Design review of the part shown in the three views and the two pictorial views. Dimensions are in mm from the part's minimum x, y and z. Coordinates: 2 decimals unless noted, no trailing zeros. Loops run counter-clockwise (first coordinate to the right, second up) from the corner with the lowest first, then second, coordinate; pieces in that order, holes last. Notation, with made-up numbers: (86.25, 74.25) -> (143.25, 74.25) arc R13 ccw to (143.25, 99.25) -> close; hole circle Ø4 at (78.5, 32). An arc over 180 degrees is marked (long way). One line per item, written item: value. Start each with the question number.
1. Draft analysis for pull direction Z (two halves, no side actions). For the marked faces 1, 2 and 3, state which applies: pulls with the +Z half, pulls with the -Z half, needs draft (parallel to the pull), parting line crosses it, or undercut.
2. Add section D-D on z = 48.5. Write out the cut boundary in (x, y).
3. Add section A-A on x = 14. Write out the cut boundary in (y, z).
4. For probe 1 along X at (y, z) = (2.5, 47.75); probe 2 along Z at (x, y) = (14, 3.15); probe 3 along X at (y, z) = (4.05, 3.5), list the stretches that pass through material, from the lowest coordinate up.
5. Insertion check: pin 1 (3 mm diameter, centred on x = 24, y = 2.5, fed in from -Z); pin 2 (3 mm diameter, centred on x = 4, y = 2.5, fed in from +Z). Each pin has a flat end and moves straight along its axis. Give the tip position at first contact, or say it passes through.
6. Add section B-B on z = 24. Write out the cut boundary in (x, y).
7. Add section C-C on y = 2.5. Write out the cut boundary in (x, z).
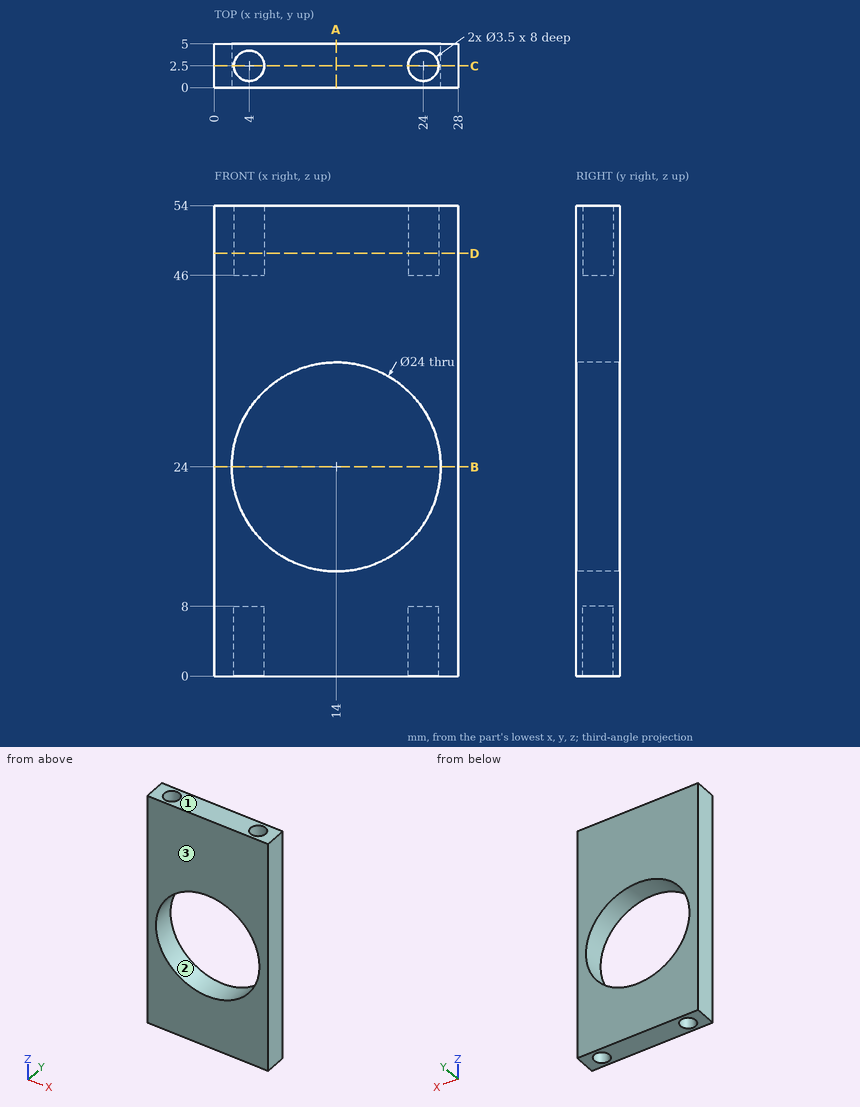
Worked answers:
1. face 1: pulls with the +Z half
1. face 2: undercut
1. face 3: needs draft
2. outline: (0, 0) -> (28, 0) -> (28, 5) -> (0, 5) -> close; hole circle Ø3.5 at (4, 2.5); hole circle Ø3.5 at (24, 2.5)
3. outline: (0, 0) -> (5, 0) -> (5, 12) -> (0, 12) -> close; (0, 36) -> (5, 36) -> (5, 54) -> (0, 54) -> close
4. probe 1: x = 0 to 2.25, 5.75 to 22.25, 25.75 to 28
4. probe 2: z = 0 to 12, 36 to 54
4. probe 3: x = 0 to 3.19, 4.81 to 23.19, 24.81 to 28
5. pin 1: stops at z = 8
5. pin 2: stops at z = 46
6. outline: (0, 0) -> (2, 0) -> (2, 5) -> (0, 5) -> close; (26, 0) -> (28, 0) -> (28, 5) -> (26, 5) -> close
7. outline: (0, 0) -> (2.25, 0) -> (2.25, 8) -> (5.75, 8) -> (5.75, 0) -> (22.25, 0) -> (22.25, 8) -> (25.75, 8) -> (25.75, 0) -> (28, 0) -> (28, 54) -> (25.75, 54) -> (25.75, 46) -> (22.25, 46) -> (22.25, 54) -> (5.75, 54) -> (5.75, 46) -> (2.25, 46) -> (2.25, 54) -> (0, 54) -> close; hole circle Ø24 at (14, 24)
